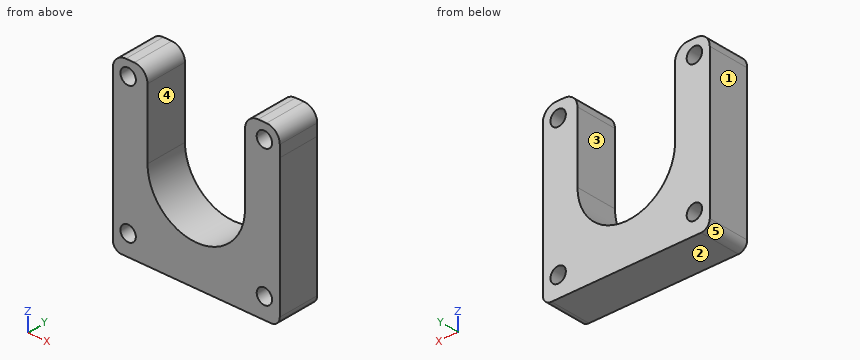
from build123d import *

# Parameters (mm, degrees)
CROQUIS1_R              = 1.75
SALIENTE_EXTRUIR1_DEPTH = 9.5


with BuildPart() as part:
    # Croquis1 → Saliente-Extruir1 (new body)
    with BuildSketch(Plane(origin=(0, 0, 0), x_dir=(1, 0, 0), z_dir=(0, 1, 0))):
        with BuildLine():
            Line((16.499992006, -9.994055242), (16.499992006, -10.627447868))
            ThreePointArc((16.499992006, -10.627447868), (15.618184374, -12.751891582), (13.491151278, -13.627434842))
            Line((13.491151278, -13.627434842), (11.591163268, -13.621835726))
            ThreePointArc((11.591163268, -13.621835726), (9.475560282, -12.740041121), (8.600003995, -10.621848752))
            Line((8.600003995, -10.621848752), (8.600003995, 5.283742))
            ThreePointArc((8.600003995, 5.283742), (-2.499996004, 16.383742), (-13.599996004, 5.283742))
            Line((-13.599996004, 5.283742), (-13.599996004, -10.538745555))
            ThreePointArc((-13.599996004, -10.538745555), (-14.481803636, -12.663189268), (-16.608836732, -13.538732529))
            Line((-16.608836732, -13.538732529), (-18.508832643, -13.533133389))
            ThreePointArc((-18.508832643, -13.533133389), (-20.624435657, -12.651338755), (-21.499991915, -10.533146335))
            Line((-21.499991915, -10.533146335), (-21.499991004, 23.50000907))
            ThreePointArc((-21.499991004, 23.50000907), (-20.914206292, 24.914222817), (-19.499993974, 25.50001098))
            Line((-19.499993974, 25.50001098), (14.499990025, 25.50001098))
            ThreePointArc((14.499990025, 25.50001098), (15.914205688, 24.914224662), (16.499992996, 23.500009))
            Line((16.499992996, 23.500009), (16.499992006, -7.988673633))
            Line((16.499992006, -7.988673633), (16.499992006, -9.994055242))
        make_face()
        with Locations(Location((-17.999996004, -10.216258, 0), (0, 0, 270))):
            Circle(CROQUIS1_R, mode=Mode.SUBTRACT)
        with Locations(Location((-17.999996004, 20.783742, 0), (0, 0, 270))):
            Circle(CROQUIS1_R, mode=Mode.SUBTRACT)
        with Locations(Location((13.000003996, -10.216258, 0), (0, 0, 270))):
            Circle(CROQUIS1_R, mode=Mode.SUBTRACT)
        with Locations(Location((13.000003996, 20.783742, 0), (0, 0, 270))):
            Circle(CROQUIS1_R, mode=Mode.SUBTRACT)
    extrude(amount=SALIENTE_EXTRUIR1_DEPTH)


solid = part.part
Source: CAD feature listing. Evaluate the final solid. Frame: model axes, mm. Face numbers are marked on the shaded views. A direction names the side the tool comes from. Coordinates: 2 decimals unless noted, no trailing zeros. Loops run counter-clockwise (first coordinate to the right, second up) from the corner with the lowest first, then second, coordinate; pieces in that order, holes last. Notation, with made-up numbers: (65, -36.75) - (100, -36.75) arc R8 cw to (100, -21.75) - close; hole circle Ø5 at (40.5, 50.5). An arc over 180 degrees is marked (long way). One line per item, written item: value. Start each with the question number.
1. Set-up query: the marked faces 4 and 5. Return all of +Z, -Z, +X, -X, +Y, -Y with unobstructed straight access to the full face (end or side cutting, diameter ignored); none if empty.
2. Section D-D (z = -8). Return the cut outline in (x, y).
3. Section B-B (z = 3). Return the cut outline in (x, y), and give its area (3 significant figures).
4. Contact query for flat-ended pins moving along their axis: P1, Ø1, axis at x = -15.5, y = 2.5, coming from the +Z side; P2, Ø5, axis at x = -12.5, y = 8, coming from the +Z side. Output: stop coordinate, or through.
5. Section C-C (z = -22). Return the cut outline in (x, y).
6. Ray query, L1, parallel to X at y = 7.5, z = -5; L2, parallel to X at y = 8.25, z = -21; L3, parallel to Z at x = -3, y = 1.5. Return the intervals inside material, ascending.
7. Section A-A (y = 7.75). Return the cut outline in (x, z).
8. Mould query, pull axis X, two halves, no side actions, for the marked faces 1, 2 and 3. Classes: pulls with the +X half, pulls with the -X half, needs draft (parallel to the pull), parting line crosses it, or undercut.
Verdict:
1. face 4: +Z, +Y, -Y
1. face 5: -Z, -X, +Y, -Y
2. outline: (-21.5, 0) - (-13.26, 0) - (-13.26, 9.5) - (-21.5, 9.5) - close; (8.26, 0) - (16.5, 0) - (16.5, 9.5) - (8.26, 9.5) - close
3. outline: (-21.5, 0) - (-13.6, 0) - (-13.6, 9.5) - (-21.5, 9.5) - close; (8.6, 0) - (16.5, 0) - (16.5, 9.5) - (8.6, 9.5) - close
3. area: 150 mm2
4. P1: stops at z = 13.48
4. P2: stops at z = 13.08
5. outline: (-21.5, 0) - (-19.26, 0) - (-19.26, 9.5) - (-21.5, 9.5) - close; (-16.74, 0) - (11.74, 0) - (11.74, 9.5) - (-16.74, 9.5) - close; (14.26, 0) - (16.5, 0) - (16.5, 9.5) - (14.26, 9.5) - close
6. L1: x = -21.5 to -13.6, 8.6 to 16.5
6. L2: x = -21.5 to -19.74, -16.26 to 11.26, 14.74 to 16.5
6. L3: z = -25.5 to -16.37
7. outline: (-21.5, -23.5) arc R2 ccw to (-19.5, -25.5) - (14.5, -25.5) arc R2 ccw to (16.5, -23.5) - (16.5, 10.63) arc R3 ccw to (13.49, 13.63) - (11.59, 13.62) arc R3 ccw to (8.6, 10.62) - (8.6, -5.28) arc R11.1 cw to (-13.6, -5.28) - (-13.6, 10.54) arc R3 ccw to (-16.61, 13.54) - (-18.51, 13.53) arc R3 ccw to (-21.5, 10.53) - close; hole circle Ø3.5 at (-18, -20.78); hole circle Ø3.5 at (-18, 10.22); hole circle Ø3.5 at (13, -20.78); hole circle Ø3.5 at (13, 10.22)
8. face 1: pulls with the -X half
8. face 2: needs draft
8. face 3: undercut
